Source: three-view drawing plus pictorial views. Frame: mm from the lowest corner of the part. A direction names the side the tool comes from. Give positions to 0.01 mm unless a question says otherwise; leave off trailing zeros. Order: outer loops, then holes, each group sorted by start corner. A loop starts at its lowest first (then second) coordinate and runs counter-clockwise, first axis right, second up. Notation, with made-up numbers: (63.25, 0.5) - (120.25, 0.5) arc R11 cw to (120.25, 6.5) - close; hole circle Ø1 at (31.25, 16.25). An arc over 180 degrees is marked (long way). Use one line per item in the form item = value.
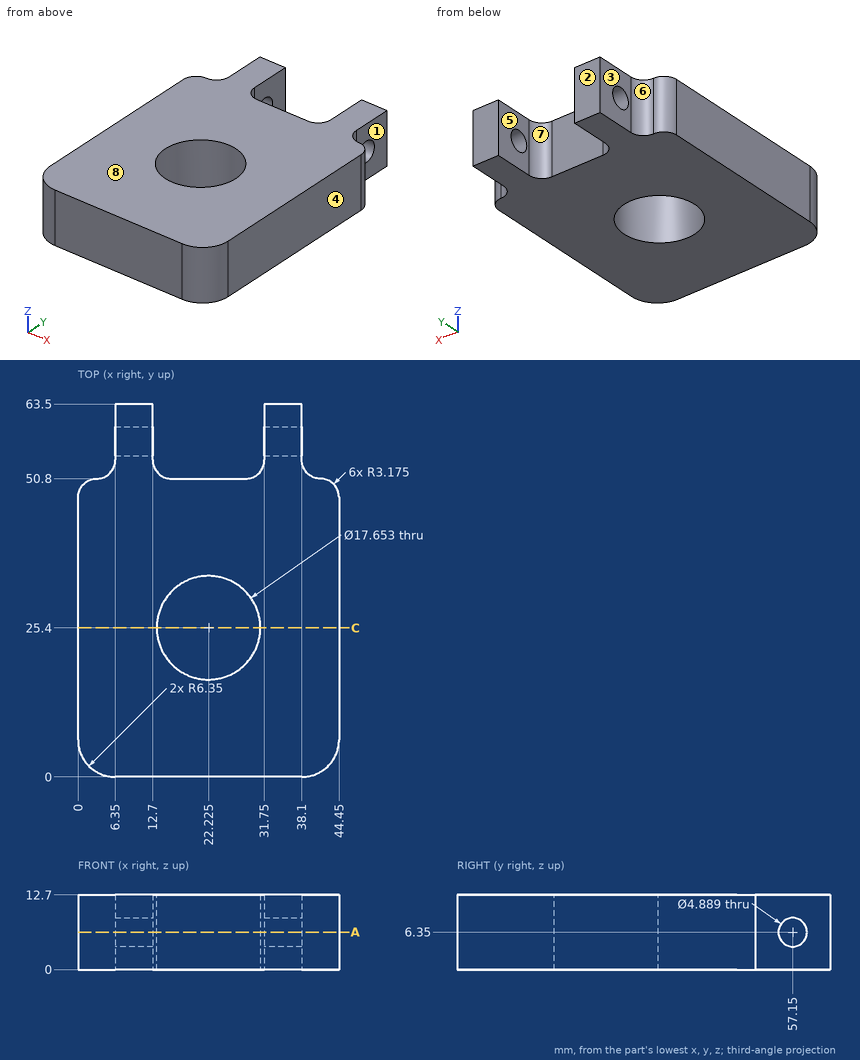
(1) Pull-direction query (X, two-part tool) for the marked faces 6, 7 and 8; classes: released by +X, released by -X, zero draft, split by the parting line, or undercut.
Computed values:
face_6 = released by -X
face_7 = undercut
face_8 = zero draft
(2) Contact query for flat-ended pins moving along their axis: pin 1 Ø6.5 at (y, z) = (57.15, 6.35) entering from -X; pin 2 Ø3 at (x, z) = (6, 1.5) entering from -Y; pin 3 Ø6.5 at (x, z) = (20.5, 6.5) entering from +Y; pin 4 Ø3 at (y, z) = (60.5, 6) entering from +X. Output: stop coordinate, or through.
Computed values:
pin_1 = 6.35
pin_2 = 0
pin_3 = 50.8
pin_4 = 38.1
(3) Ray query, line 1 along Y through (x, z) = (11.5, 6.35) (1 decimal); line 2 along Z through (x, y) = (34, 57); line 3 along X through (y, z) = (58.5, 11). Return the intervals inside material, ascending.
Computed values:
line_1 = 0 to 54.7, 59.6 to 63.5
line_2 = 0 to 3.91, 8.79 to 12.7
line_3 = 6.35 to 12.7, 31.75 to 38.1
(4) Cut plane A-A on z = 6.35. Give the number of separate pieces and of enclosed holes in the cut face, plus the area to 3 significant figures.
Computed values:
separate_pieces = 3
enclosed_holes = 1
area = 2,100 mm²
(5) Cut plane C-C on y = 25.4. Output: boundary loops of the cut face in (x, z).
Computed values:
outline = (0, 0) - (13.4, 0) - (13.4, 12.7) - (0, 12.7) - close; (31.05, 0) - (44.45, 0) - (44.45, 12.7) - (31.05, 12.7) - close
(6) Reachability of the marked faces 1, 2, 3, 4 and 5 from +Z, -Z, +X, -X, +Y, -Y: full face, straight path, thin tool, end or side. Return the list, or none.
Computed values:
face_1 = +Z, -Z, +X, +Y
face_2 = +Z, -Z, +X, -X, +Y
face_3 = +Z, -Z, -X, +Y
face_4 = +Z, -Z, +X, +Y, -Y
face_5 = +Z, -Z, +Y
